```python
from build123d import *

# Parameters (mm, degrees)
F1_DEPTH = 76.2
F2_R     = 5.08
F3_R     = 5.08


with BuildPart() as f1:
    # F0 (on Front) → F1 (new body)
    with BuildSketch(Plane.XZ):
        Polygon((-40.24671, 7.053584), (37.549719, 19.293554), (-52.071765, 19.293554), align=None)
    extrude(amount=F1_DEPTH)

    # F2
    f2_edges = [f1.edges().sort_by_distance(p)[0] for p in [
        (-7.261023, -76.2, 19.293554),
    ]]
    fillet(f2_edges, radius=F2_R)

    # F3
    f3_edges = [f1.edges().sort_by_distance(p)[0] for p in [
        (-7.261023, 0, 19.293554),
    ]]
    fillet(f3_edges, radius=F3_R)


solid = f1.part
```
Read the model definition and answer for the solid it produces. Units are mm, in the model's axes. Round coordinates to 2 decimals unless told otherwise and drop trailing zeros. Loops run counter-clockwise (first coordinate to the right, second up) from the corner with the lowest first, then second, coordinate; pieces in that order, holes last. Notation, with made-up numbers: (-27.75, -8.5) -> (-21.75, -8.5) arc R31 ccw to (-21.75, 25.5) -> close; hole circle Ø9 at (38.5, 77). An arc over 180 degrees is marked (long way). One line per item, written item: value.
1) A cutting plane is placed at B-B (y = -64). Determine the outline of the cut face in (x, z), and give its area (3 significant figures).
Answer list:
outline: (-52.07, 19.29) -> (-40.25, 7.05) -> (37.55, 19.29) -> close
area: 548 mm²
2) A cutting plane is placed at D-D (x = -11). Determine the outline of the cut face in (y, z).
Answer list:
outline: (-76.2, 11.66) -> (0, 11.66) -> (0, 14.21) arc R5.08 ccw to (-5.08, 19.29) -> (-71.12, 19.29) arc R5.08 ccw to (-76.2, 14.21) -> close
3) Consider L1, parallel to Y at x = -39.5, z = 18.5; L2, parallel to Z at x = 11.5, y = -12.5; L3, parallel to Y at x = 6, z = 16. Determine where each line is inside the solid, lowest interval first. Write a range as [from, to].
Answer list:
L1: y = [-73.85, -2.35]
L2: z = [15.2, 19.29]
L3: y = [-75.88, -0.32]
4) A cutting plane is placed at A-A (x = -25.5). Determine the outline of the cut face in (y, z).
Answer list:
outline: (-76.2, 9.37) -> (0, 9.37) -> (0, 14.21) arc R5.08 ccw to (-5.08, 19.29) -> (-71.12, 19.29) arc R5.08 ccw to (-76.2, 14.21) -> close
5) A flat-ended cylindrical pin translates along its axis: P1, Ø10, axis at x = -28, y = -66, coming from the -Z side. Find the tip coordinate at first contact, or state that the pin passes through.
Answer list:
P1: stops at z = 8.19
6) A cutting plane is placed at C-C (z = 11.5). Determine the outline of the cut face in (x, y).
Answer list:
outline: (-44.54, -76.2) -> (-11.99, -76.2) -> (-11.99, 0) -> (-44.54, 0) -> close
